Source: CAD feature listing. Evaluate the final solid. Frame: model axes, mm. Face numbers are marked on the shaded views. A direction names the side the tool comes from. Give positions to 0.01 mm unless a question says otherwise; leave off trailing zeros. Loops run counter-clockwise (first coordinate to the right, second up) from the corner with the lowest first, then second, coordinate; pieces in that order, holes last.
```python
from build123d import *

# Parameters (mm, degrees)
SKETCH_1_W          = 264.89
SKETCH_1_H          = 5
SKETCH_2_R          = 14.5
EXTRUDE_1_DEPTH     = 23
SKETCH_3_R          = 14.5
EXTRUDE_2_DEPTH     = 23
SKETCH_4_R          = 14.5
EXTRUDE_3_DEPTH     = 23
SKETCH_5_R          = 14.5
EXTRUDE_4_DEPTH     = 23
SKETCH_7_R          = 5
CUT_EXTRUDE_1_DEPTH = 20.12
SKETCH_8_R          = 7
EXTRUDE_6_DEPTH     = 4


with BuildPart() as part:
    # 草圖1 → 旋轉1 (revolve)
    with BuildSketch(Plane.XY, mode=Mode.PRIVATE) as revolve_1_sk:
        with Locations((-132.445, 2.5)):
            Rectangle(SKETCH_1_W, SKETCH_1_H)
    revolve(revolve_1_sk.sketch.rotate(Axis((0, 0, 0), (-1, 0, 0)), 90), axis=Axis((0, 0, 0), (-1, 0, 0)))

    # 草圖2 → 填料-伸長1 (add)
    with BuildSketch(Plane.ZY.offset(240.89)):
        with Locations(Location((0, 9.5, 0), (0, 0, 270))):
            Circle(SKETCH_2_R)
    extrude(amount=-EXTRUDE_1_DEPTH)

    # 草圖3 → 填料-伸長2 (add)
    with BuildSketch(Plane.ZY.offset(192.89)):
        with Locations(Location((0, -9.5, 0), (0, 0, 90))):
            Circle(SKETCH_3_R)
    extrude(amount=-EXTRUDE_2_DEPTH)

    # 草圖4 → 填料-伸長3 (add)
    with BuildSketch(Plane.ZY.offset(144.89)):
        with Locations(Location((0, 9.5, 0), (0, 0, 270))):
            Circle(SKETCH_4_R)
    extrude(amount=-EXTRUDE_3_DEPTH)

    # 草圖5 → 填料-伸長4 (add)
    with BuildSketch(Plane.ZY.offset(96.89)):
        with Locations(Location((0, -9.5, 0), (0, 0, 90))):
            Circle(SKETCH_5_R)
    extrude(amount=-EXTRUDE_4_DEPTH)

    # 草圖7 → 除料-伸長1 (cut)
    with BuildSketch(Plane(origin=(0, 0, 0), x_dir=(0, 0, -1), z_dir=(1, 0, 0))):
        Circle(SKETCH_7_R)
    extrude(amount=-CUT_EXTRUDE_1_DEPTH, mode=Mode.SUBTRACT)

    # 草圖8 → 填料-伸長6 (add)
    with BuildSketch(Plane(origin=(-20.12, 0, 0), x_dir=(0, 0, -1), z_dir=(1, 0, 0))):
        Circle(SKETCH_8_R)
    extrude(amount=-EXTRUDE_6_DEPTH)


solid = part.part
```
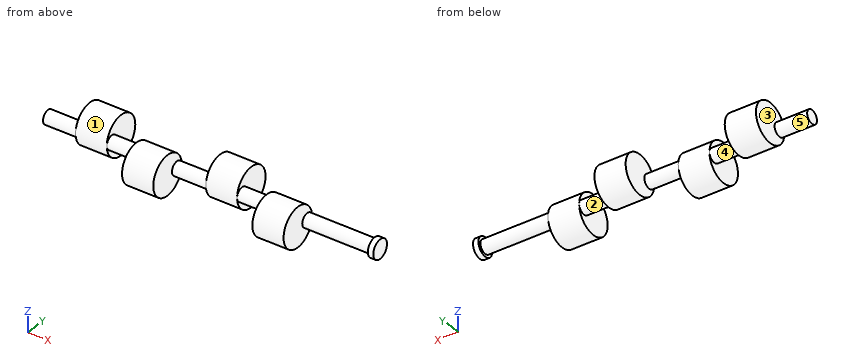
(1) First-contact query: pin 1 (4 mm diameter, centred on x = -99.5, z = -6, fed in from +Y); pin 2 (12 mm diameter, centred on x = -106, z = 5, fed in from +Y); pin 3 (8.5 mm diameter, centred on y = 9, z = -7, fed in from -X); pin 4 (14.5 mm diameter, centred on y = -5, z = -6.5, fed in from -X). Flat tips, straight axial feed; report the tip coordinate or a pass-through.
A:
pin 1: stops at y = 3
pin 2: stops at y = 5
pin 3: stops at x = -240.89
pin 4: stops at x = -264.89
(2) Section B-B, the plane z = -10.25. Return the cut outline in (x, y).
A:
outline: (-240.89, -0.76) - (-217.89, -0.76) - (-217.89, 19.76) - (-240.89, 19.76) - close; (-192.89, -19.76) - (-169.89, -19.76) - (-169.89, 0.76) - (-192.89, 0.76) - close; (-144.89, -0.76) - (-121.89, -0.76) - (-121.89, 19.76) - (-144.89, 19.76) - close; (-96.89, -19.76) - (-73.89, -19.76) - (-73.89, 0.76) - (-96.89, 0.76) - close
(3) Mould query, pull axis X, two halves, no side actions, for the marked faces 3, 4 and 5. Classes: pulls with the +X half, pulls with the -X half, needs draft (parallel to the pull), parting line crosses it, or undercut.
A:
face 3: pulls with the -X half
face 4: undercut
face 5: needs draft
(4) Section A-A, the plane y = -9.5. Return the cut outline in (x, z), then the cut area to 3 significant figures.
A:
outline: (-192.89, -14.5) - (-169.89, -14.5) - (-169.89, 14.5) - (-192.89, 14.5) - close; (-96.89, -14.5) - (-73.89, -14.5) - (-73.89, 14.5) - (-96.89, 14.5) - close
area: 1,330 mm2
(5) Section C-C, the plane y = 20. Return the cut outline in (x, z).
A:
outline: (-240.89, -10) - (-217.89, -10) - (-217.89, 10) - (-240.89, 10) - close; (-144.89, -10) - (-121.89, -10) - (-121.89, 10) - (-144.89, 10) - close
(6) Ray query, line 1 along X through (y, z) = (-5.5, -3); line 2 along X through (y, z) = (-14, 2.25); line 3 along X through (y, z) = (22, -5). Return the intervals inside material, ascending.
A:
line 1: x = -192.89 to -169.89, -96.89 to -73.89, -24.12 to -20.12
line 2: x = -192.89 to -169.89, -96.89 to -73.89
line 3: x = -240.89 to -217.89, -144.89 to -121.89
(7) Reachability of the marked faces 1 and 2 from +Z, -Z, +X, -X, +Y, -Y: full face, straight path, thin tool, end or side. Return the list, or none.
A:
face 1: -X
face 2: none
(8) Section D-D, the plane x = -151.5. Return the cut outline in (y, z), then the cut area to 3 significant figures.
A:
outline: circle Ø10 at (0, 0)
area: 78.5 mm2
